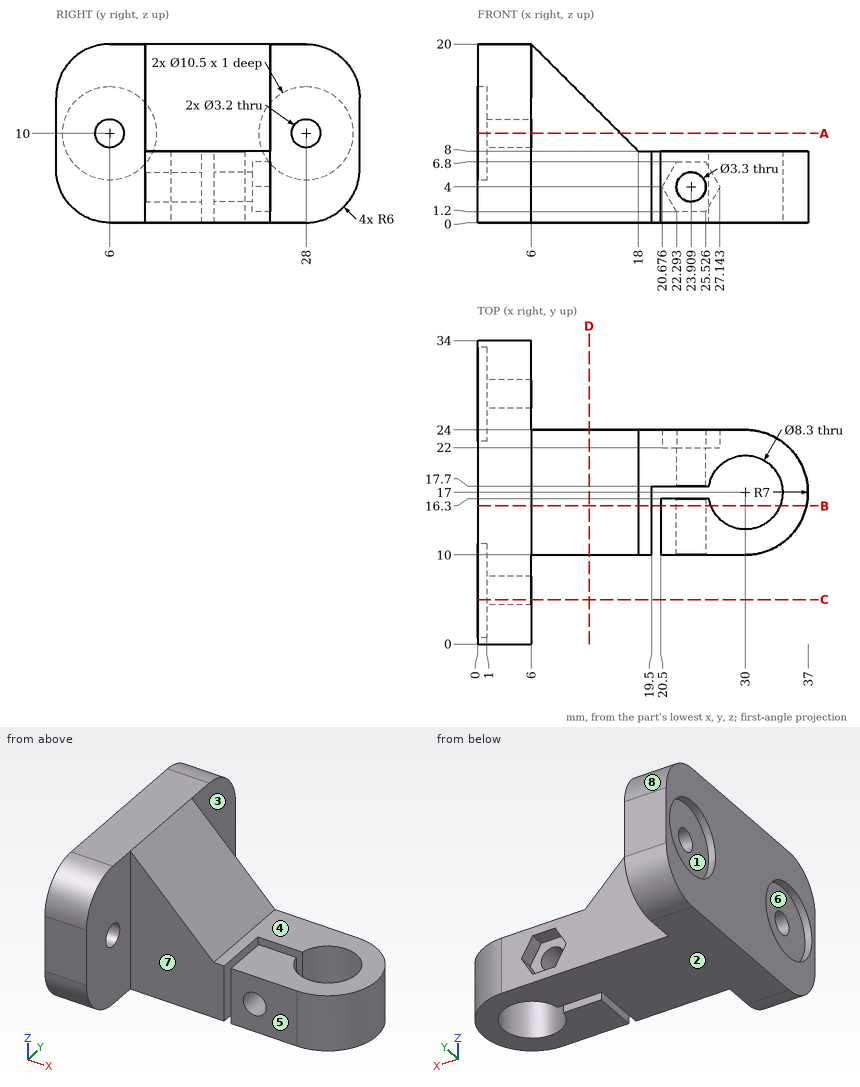
Source: three-view drawing plus pictorial views. Frame: mm from the lowest corner of the part. A direction names the side the tool comes from. Give positions to 0.01 mm unless a question says otherwise; leave off trailing zeros. Order: outer loops, then holes, each group sorted by start corner. A loop starts at its lowest first (then second) coordinate and runs counter-clockwise, first axis right, second up. Notation, with made-up numbers: (51.5, 35) -> (98.5, 35) arc R19 ccw to (98.5, 65) -> close; hole circle Ø5 at (53.5, -32). An arc over 180 degrees is marked (long way). Write each question's results on one line, items separated by ' | '. Start each with the question number.
Item 1: Cut plane B-B on y = 15.5. Return the cut outline in (x, z), then the cut area to 3 significant figures.
Item 2: Line query: line 1 (Y direction, x = 3, z = 9.25) (1 decimal); line 2 (Y direction, x = 30, z = 3.25); line 3 (X direction, y = 5.5, z = 6). Output: solid intervals per line, ascending.
Item 3: Mould query, pull axis Z, two halves, no side actions, for the marked faces 6, 7 and 8. Classes: pulls with the +Z half, pulls with the -Z half, needs draft (parallel to the pull), parting line crosses it, or undercut.
Item 4: Set-up query: the marked faces 1, 2, 3, 4 and 5. Return all of +Z, -Z, +X, -X, +Y, -Y with unobstructed straight access to the full face (end or side cutting, diameter ignored); none if empty.
Item 5: Cut plane D-D on x = 12.5. Return the cut outline in (y, z).
Item 6: Cut plane C-C on y = 5. Return the cut outline in (x, z).
Item 7: Contact query for flat-ended pins moving along their axis: P1, Ø1, axis at x = 24.5, y = 23, coming from the +Z side; P2, Ø10, axis at x = 17.5, z = 12, coming from the -Y side; P3, Ø8, axis at y = 30.5, z = 10, coming from the +X side; P4, Ø7.5, axis at x = 30, y = 17, coming from the +Z side. Output: stop coordinate, or through.
Item 8: Cut plane A-A on z = 10. Return the cut outline in (x, y).
Established:
1) outline: (0, 0) -> (19.5, 0) -> (19.5, 8) -> (18, 8) -> (6, 20) -> (0, 20) -> close; (20.5, 0) -> (26.13, 0) -> (26.13, 8) -> (20.5, 8) -> close; (33.87, 0) -> (36.84, 0) -> (36.84, 8) -> (33.87, 8) -> close; hole circle Ø3.3 at (23.91, 4) | area: 360 mm^2
2) line 1: 0 to 4.6, 7.4 to 26.6, 29.4 to 34 | line 2: 10 to 12.85, 21.15 to 24 | line 3: 1 to 6
3) face 6: undercut | face 7: needs draft | face 8: pulls with the +Z half
4) face 1: -X | face 2: -Z, +X, -X, +Y, -Y | face 3: +Z, -Z, +X, +Y | face 4: +Z, +X, +Y, -Y | face 5: +Z, -Z, +X, -Y
5) outline: (10, 0) -> (24, 0) -> (24, 13.5) -> (10, 13.5) -> close
6) outline: (0, 0.08) -> (6, 0.08) -> (6, 8.75) -> (1, 8.75) -> (1, 4.85) -> (0, 4.85) -> close; (0, 15.15) -> (1, 15.15) -> (1, 11.25) -> (6, 11.25) -> (6, 19.92) -> (0, 19.92) -> close
7) P1: z = 8 | P2: y = 10 | P3: x = 6 | P4: through
8) outline: (0, 0) -> (6, 0) -> (6, 4.4) -> (1, 4.4) -> (1, 0.75) -> (0, 0.75) -> close; (0, 11.25) -> (1, 11.25) -> (1, 7.6) -> (6, 7.6) -> (6, 10) -> (16, 10) -> (16, 24) -> (6, 24) -> (6, 26.4) -> (1, 26.4) -> (1, 22.75) -> (0, 22.75) -> close; (0, 33.25) -> (1, 33.25) -> (1, 29.6) -> (6, 29.6) -> (6, 34) -> (0, 34) -> close
